Input: part model. Units: mm. Frame: model coordinates. A direction names the side the tool comes from. Coordinates: 2 decimals unless noted, no trailing zeros. Order: outer loops, then holes, each group sorted by start corner. A loop starts at its lowest first (then second) coordinate and runs counter-clockwise, first axis right, second up. Notation, with made-up numbers: (24.5, 35) - (54.5, 35) arc R23 cw to (54.5, 55) - close; hole circle Ø2 at (89.25, 52). An arc over 180 degrees is marked (long way). Answer as CSV lines item,"result". Start each with the question number.
Item 1: Section A-A (y = 0). Output: boundary loops of the cut face in (x, z), and give its area (3 significant figures).
Item 2: Access query for faces 1 (the cylindrical face through (49.3, 47.69, -15.02)), 2 (the flat face through (54, 25, -78)), 3 (the cylindrical face through (25.787, -119.884, 5.276)). Directions: +Z, -Z, +X, -X, +Y, -Y. A direction counts if a zero-diameter tool reaches every point of the face in a straight line with its end or side. Return the directions, or none.
Item 3: First-contact query: pin 1 (1 mm diameter, centred on x = 70.5, z = 109, fed in from +Y); pin 2 (4 mm diameter, centred on x = 34, z = 50.5, fed in from +Y); pin 3 (6 mm diameter, centred on x = 49, z = 57, fed in from -Y); pin 4 (1.5 mm diameter, centred on y = 50, z = 56.5, fed in from -X). Flat tips, straight axial feed; report the tip coordinate or a pass-through.
Item 4: Section D-D (z = 86.5). Output: boundary loops of the cut face in (x, y).
Item 5: Section C-C (x = 37). Output: boundary loops of the cut face in (y, z), and give its area (3 significant figures).
Item 6: Material intervals for line 1 along Z through (x, y) = (74.5, 0); line 2 along Z through (x, y) = (49, 0); line 3 along Y through (x, z) = (14.5, -44), sorted ascending.
Item 7: Draft query along Z for faces 4 (the cylindrical face through (76.68, -17.34, 78.1)), 5 (the flat face through (95, -54, 108)), 6 (the cylindrical face through (50.63, 138.304, 43.554)), 7 (the cylindrical face through (22.68, -17.34, 78.1)). Return one class per face: +Z half, -Z half, draft (parallel to the pull), parting line (faces both ways), or undercut.
Autodesk Inventor part; units mm, degrees
ref_plane "XZ Plane" through (0, 0, 0) normal (0, 1, 0) x (-1, 0, 0)
sketch "Sketch1" plane through (0, 0, 0) normal (1, 0, 0) x (0, 1, 0)
  circle A0 centre (0, 0) radius 50
  circle A1 centre (0, 0) radius 80
  dimension "d0" = 100
  dimension "d1" = 160
extrude "Extrusion1" add sketch "Sketch1" along normal blind 100
ref_plane "Work Plane1" through (0, 0, 0) normal (0, 0, 1) x (1, 0, 0)
sketch "Sketch2" plane through (0, 0, 0) normal (0, 0, 1) x (1, 0, 0)
  line L0 (0, 80) -> (100, 80)
  line L1 (54, 80) -> (54, 120)
  line L2 (54, 120) -> (46, 120)
  line L3 (46, 120) -> (46, 80)
  line L4 (0, -80) -> (0, 80)
  line L5 (-20, 0) -> (120, 0)
  point P0 (0, 0)
  dimension "d5" = 8
  dimension "d6" = 46
  dimension "d7" = 40
revolve "Revolution1" add sketch "Sketch2" angle 360 about axis through (-10, 0, 0) along (1, 0, 0)
ref_plane "Work Plane2" through (50, 0, 0) normal (1, 0, 0) x (0, 1, 0)
sketch "Sketch4" plane through (50, 0, 0) normal (1, 0, 0) x (0, 1, 0)
  circle A0 centre (0, 0) radius 145
  circle A1 centre (0, 0) radius 120
  dimension "d12" = 290
  dimension "d13" = 240
extrude "Extrusion2" add sketch "Sketch4" along normal mid plane 90
sketch "Sketch5" plane through (95, 0, 0) normal (1, 0, 0) x (0, 0, -1)
  point P0 (0, 0)
properties part number "DiscoPaleSatdio1-3"
Determined:
1,outline,"(0, -80) - (46, -80) - (46, -120) - (5, -120) - (5, -145) - (95, -145) - (95, -120) - (54, -120) - (54, -80) - (100, -80) - (100, -50) - (0, -50) - close; (0, 50) - (100, 50) - (100, 80) - (54, 80) - (54, 120) - (95, 120) - (95, 145) - (5, 145) - (5, 120) - (46, 120) - (46, 80) - (0, 80) - close"
1,area,"11,100 mm^2"
2,face 1,"+X, -X"
2,face 2,"+X"
2,face 3,"-X"
3,pin 1,"stops at y = 96.19"
3,pin 2,"stops at y = 136.65"
3,pin 3,"stops at y = -134.57"
3,pin 4,"stops at x = 0"
4,outline,"(5, -116.37) - (95, -116.37) - (95, -83.17) - (54, -83.17) - (54, 83.17) - (95, 83.17) - (95, 116.37) - (5, 116.37) - (5, 83.17) - (46, 83.17) - (46, -83.17) - (5, -83.17) - close"
5,outline,"circle Ø290 at (0, 0); circle Ø160 at (0, 0); hole circle Ø240 at (0, 0); hole circle Ø100 at (0, 0)"
5,area,"33,100 mm^2"
6,line 1,"z = -145 to -120, -80 to -50, 50 to 80, 120 to 145"
6,line 2,"z = -145 to -50, 50 to 145"
6,line 3,"y = -138.16 to -111.64, -66.81 to -23.75, 23.75 to 66.81, 111.64 to 138.16"
7,face 4,"undercut"
7,face 5,"draft"
7,face 6,"parting line"
7,face 7,"undercut"
